from build123d import *

# Parameters (mm, degrees)
F0_W            = 20
F0_H            = 20
F1_DEPTH        = 463
F2_R            = 2.1
F3_DEPTH        = 463.001
F4_R            = 1
F6_DEPTH        = 463.001
F6_COPIES_COUNT = 4


# Not quite as in the source:
# - a pattern or mirror of a feature is missing from the dataset's text; its kind, count and spacing are read off the source's solid


with BuildPart() as f1:
    # F0 (on Front) → F1 (new body)
    with BuildSketch(Plane.XZ):
        Rectangle(F0_W, F0_H)
    extrude(amount=F1_DEPTH)

    # F2 (on face) → F3 (cut, through all)
    with BuildSketch(Plane.XZ.offset(463)):
        Circle(F2_R)
    extrude(amount=-F3_DEPTH, mode=Mode.SUBTRACT)

    # F4
    f4_edges = [f1.edges().sort_by_distance(p)[0] for p in [
        (-10, -231.5, 10),
        (10, -231.5, 10),
        (10, -231.5, -10),
        (-10, -231.5, -10),
    ]]
    fillet(f4_edges, radius=F4_R)

    # F5 (on face) → F6 (cut, through all)
    with BuildSketch(Plane.XZ.offset(463)):
        Polygon((0, 3.9006601718), (0, 10), (-2.84, 10), (-4.64, 10), (-2.84, 8.2), (-5.4993398282, 8.2), (-5.4993398282, 6.56), (-2.84, 3.9006601718), align=None)
        Polygon((-6.5693398282, 8.2), (-8.2, 8.2), (-7.0953059148, 7.0953059148), (-6.5693398282, 7.6212720014), align=None)
    f6 = extrude(amount=-F6_DEPTH, mode=Mode.SUBTRACT)

    # F6_copies: F6 ×4 about axis
    f6_copies_axis = Axis((0, 0, 0), (0, 1, 0))
    for i in range(1, F6_COPIES_COUNT):
        add(f6.rotate(f6_copies_axis, i * 360 / F6_COPIES_COUNT), mode=Mode.SUBTRACT)

    # F6_copies1: F6 across plane
    add(f6.mirror(Plane(origin=(0, 0, 0), x_dir=(-0.7071067812, 0, -0.7071067812), z_dir=(0.7071067812, 0, -0.7071067812))), mode=Mode.SUBTRACT)

    # F6_copies2: F6 across plane
    add(f6.mirror(Plane(origin=(0, 0, 0), x_dir=(-1, 0, 0), z_dir=(0, 0, -1))), mode=Mode.SUBTRACT)

    # F6_copies3: F6 across plane
    add(f6.mirror(Plane(origin=(0, 0, 0), x_dir=(0, 0, 1), z_dir=(1, 0, 0))), mode=Mode.SUBTRACT)

    # F6_copies4: F6 across plane
    add(f6.mirror(Plane(origin=(0, 0, 0), x_dir=(0.7071067812, 0, -0.7071067812), z_dir=(-0.7071067812, 0, -0.7071067812))), mode=Mode.SUBTRACT)


solid = f1.part
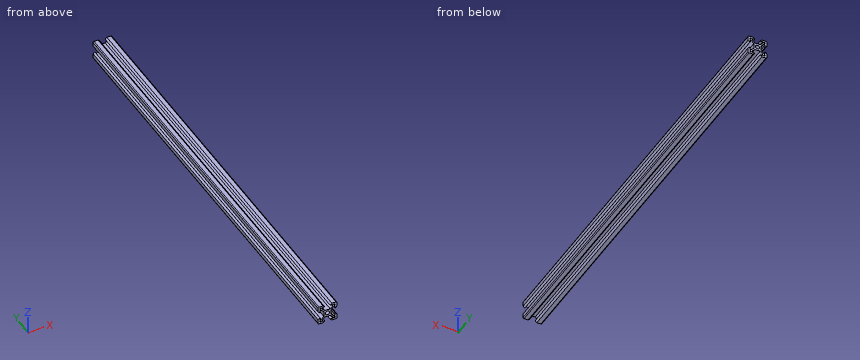
Could you check a few things on this model? Use its own coordinates, in mm. Round coordinates to 2 decimals unless told otherwise and drop trailing zeros. Write item = value, one per line.
1) I need wall thicknesses on line 1 along Z through (x, y) = (7.75, -97); line 2 along Z through (x, y) = (-4, -116). Which ranges of each line are inside material? Lowest first, please. Write a range as from..to.
Computed:
line_1 = -10..-8.2, -6.57..-5.5, 5.5..6.57, 8.2..10
line_2 = -9.36..-8.2, -5.06..-2.94, 2.94..5.06, 8.2..9.36
2) Imagine slicing it at A-A (y = -416). Give the number of separate pieces and of enclosed holes in the cut face, and give its area (3 significant figures).
Computed:
separate_pieces = 1
enclosed_holes = 5
area = 162 mm2
3) I'm going to push flat-ended pins straight in: P1, Ø2, axis at y = -356.5, z = 1, coming from the -X side; P2, Ø3, axis at x = 2, y = -167, coming from the +Z side; P3, Ø4, axis at y = -232, z = -2, coming from the -X side. Where does each tip first touch, or does it pass through?
Computed:
P1 = -3.9
P2 = 8.86
P3 = -9.36
